For this review, take the finished solid that the model builds, in its own axes (mm). Give positions to 0.01 mm unless a question says otherwise; leave off trailing zeros. Write each loop counter-clockwise with the first axis right and the second up, starting at its lowest first coordinate (ties: lowest second). Pieces come first, ordered by that corner, then holes.
1) We need section C-C on x = 4.75. Give the boundary of the cut face in (y, z), and give its area (3 significant figures).
2) For P1, Ø1.5, axis at x = 0.5, z = 62, coming from the -Y side; P2, Ø2, axis at x = -5, z = 26.5, coming from the -Y side; P3, Ø1.8, axis at x = 0, y = -0.6, coming from the -Z side; P4, Ø2.5, axis at x = 0, z = 35.5, coming from the +Y side, all flat-tipped, find the tip position at first contact; note any pin that passes through.
3) We need section A-A on z = 35.5. Give the boundary of the cut face in (x, y).
4) We need section D-D on y = 1.25. Give the boundary of the cut face in (x, z).
5) We need section B-B on z = 45. Give the boundary of the cut face in (x, y).
6) Wall thickness on line 1 along Y through (x, z) = (0, 60.05) (3 decimals); line 2 along X through (y, z) = (-0.75, 54); line 3 along Z through (x, y) = (-1, -1): over which ranges is each line inside the solid? List them lowest first.
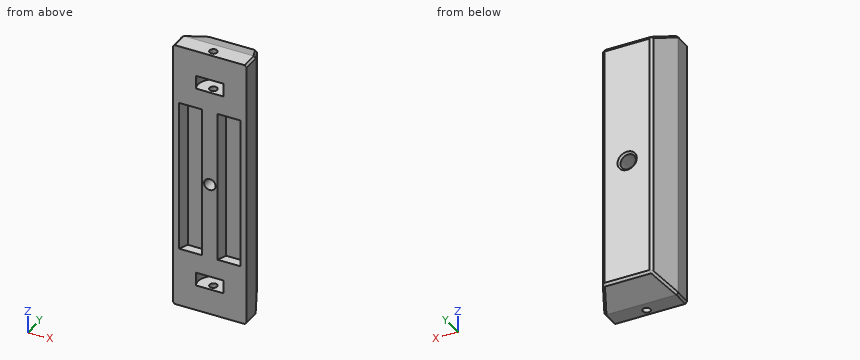
from build123d import *

# Parameters (mm, degrees)
EXTRUDE_1_DEPTH     = 71
CUT_EXTRUDE_1_DEPTH = 75.103710772
SKETCH_3_W          = 18.218739558
SKETCH_3_H          = 4.354088086
EXTRUDE_3_DEPTH     = 15.5
SKETCH_4_R          = 0.995
CUT_EXTRUDE_2_DEPTH = 12
SKETCH_5_W          = 4
SKETCH_5_H          = 3.5
SKETCH_6_R          = 1.5
CUT_EXTRUDE_3_DEPTH = 73.548604312
SKETCH_7_R          = 2.01
CUT_EXTRUDE_4_DEPTH = 5
CHAMFER_2_SIZE      = 0.5


with BuildPart() as part:
    # ｽｹｯﾁ1 → ﾎﾞｽ - 押し出し1 (new body)
    with BuildSketch(Plane.XY):
        Polygon((-6.990630221, 0), (-3.009369779, 0), (-1.990630221, -2.4), (1.990630221, -2.4), (3.009369779, 0), (6.990630221, 0), (8.009369779, -2.4), (9.609369779, -2.4), (9.609369779, 2), (6.345216172, 9), (-6.345216172, 9), (-9.609369779, 2), (-9.609369779, -2.4), (-8.009369779, -2.4), align=None)
    extrude(amount=EXTRUDE_1_DEPTH)

    # ｽｹｯﾁ2 → ｶｯﾄ - 押し出し1 (cut, through all)
    with BuildSketch(Plane(origin=(9.609369779, 0, 0), x_dir=(0, 0, -1), z_dir=(1, 0, 0))):
        Polygon((-71, 2), (-67.735846393, 9), (-71, 9), align=None)
        Polygon((-3.264153607, 9), (0, 9), (0, 2), align=None)
    extrude(amount=-CUT_EXTRUDE_1_DEPTH, mode=Mode.SUBTRACT)

    # 面取り1
    # the kernel refuses this chamfer: 0.5 mm, written as the material it takes off along each edge
    with BuildSketch(Plane(origin=(-6.138482875, 8.697897404, 3.470886905), x_dir=(0.1959067162203001, 0.5268881046463136, 0.8270486586180973), z_dir=(-0.41632572739388224, 0.8082980746110386, -0.4163257273938792)), Plane(origin=(6.138482875, 8.697897404, 3.470886905), x_dir=(-0.8270486586180952, 0.5268881046463165, 0.19590671622030123), z_dir=(0.4163257273938833, 0.8082980746110385, -0.41632572739387846))) as chamfer_1_piece_1:
        Polygon((-0.400884159, 0.228990916), (0.459173014, 0.228990916), (-0.058288855, -0.457981831), align=None)
    extrude(amount=0.4579583, mode=Mode.SUBTRACT)
    with BuildSketch(Plane(origin=(-6.138482875, 8.697897404, 67.529113095), x_dir=(-0.19590671622031064, -0.5268881046463169, 0.8270486586180926), z_dir=(-0.416325727393884, 0.808298074611038, 0.41632572739387863))) as chamfer_1_piece_2:
        Polygon((-0.459173014, 0.228990916), (0.400884159, 0.228990916), (0.058288855, -0.457981831), align=None)
    extrude(amount=0.4579583, mode=Mode.SUBTRACT)
    with BuildSketch(Plane(origin=(6.138482875, 8.697897404, 67.529113095), x_dir=(-0.8270486586180955, 0.5268881046463167, -0.19590671622029923), z_dir=(0.4163257273938827, 0.8082980746110371, 0.4163257273938819))) as chamfer_1_piece_3:
        Polygon((-0.400884159, -0.228990916), (0.459173014, -0.228990916), (-0.058288855, 0.457981831), align=None)
    extrude(amount=0.4579583, mode=Mode.SUBTRACT)
    with BuildSketch(Plane(origin=(9.609369779, -3.685841494, 71), x_dir=(-0.999621916911297, 0, 0.0274958766105822), z_dir=(0, 1, 0)), Plane(origin=(-9.609369779, 3.285841494, 71), x_dir=(0.999621916911297, 0, 0.0274958766105822), z_dir=(0, -1, 0))) as chamfer_1_piece_4:
        with BuildLine():
            Line((0.514336598, 0), (-0.028273577, -0.513558897))
            Line((-0.028273577, -0.513558897), (-0.038269797, -0.513283938))
            ThreePointArc((-0.038269797, -0.513283938), (-0.017064614, -0.256698915), (-0.009996219, 0.000274959))
            Line((-0.009996219, 0.000274959), (0.000274959, 0.009996219))
            ThreePointArc((0.000274959, 0.009996219), (0.257248832, 0.002927825), (0.514611556, 0.009996219))
            Line((0.514611556, 0.009996219), (0.514336598, 0))
        make_face()
    extrude(amount=6.971682988, mode=Mode.SUBTRACT)
    with BuildSketch(Plane(origin=(-9.609369779, 3.285841494, 0), x_dir=(0.9996219169112968, 0, -0.02749587661058639), z_dir=(0, -1, 0)), Plane(origin=(9.609369779, -3.685841494, 0), x_dir=(-0.9996219169112968, 0, -0.02749587661058639), z_dir=(0, 1, 0))) as chamfer_1_piece_5:
        with BuildLine():
            Line((0.514336598, 0), (-0.028273577, 0.513558897))
            Line((-0.028273577, 0.513558897), (-0.038269797, 0.513283938))
            ThreePointArc((-0.038269797, 0.513283938), (-0.017064614, 0.256698915), (-0.009996219, -0.000274959))
            Line((-0.009996219, -0.000274959), (0.000274959, -0.009996219))
            ThreePointArc((0.000274959, -0.009996219), (0.257248832, -0.002927825), (0.514611556, -0.009996219))
            Line((0.514611556, -0.009996219), (0.514336598, 0))
        make_face()
    extrude(amount=6.971682988, mode=Mode.SUBTRACT)
    with BuildSketch(Plane(origin=(-6.345216172, 9, 1.971704795), x_dir=(-0.441365564598093, -0.897327386401979, 0), z_dir=(0, 0, 1))) as chamfer_1_piece_6:
        with BuildLine():
            Line((0.516979525, 0), (-0.237770334, 0.459056747))
            Line((-0.237770334, 0.459056747), (-0.246743608, 0.454643091))
            ThreePointArc((-0.246743608, 0.454643091), (-0.123037104, 0.227486173), (-0.008973274, -0.004413656))
            Line((-0.008973274, -0.004413656), (0.000207861, -0.009997839))
            ThreePointArc((0.000207861, -0.009997839), (0.25858594, -0.004626004), (0.517187386, -0.009997839))
            Line((0.517187386, -0.009997839), (0.516979525, 0))
        make_face()
    extrude(amount=67.056590409, mode=Mode.SUBTRACT)
    with BuildSketch(Plane(origin=(6.345216172, 9, 1.971704795), x_dir=(0.441365564598093, -0.897327386401979, 0), z_dir=(0, 0, 1))) as chamfer_1_piece_7:
        with BuildLine():
            Line((0.516979525, 0), (-0.237770334, -0.459056747))
            Line((-0.237770334, -0.459056747), (-0.246743608, -0.454643091))
            ThreePointArc((-0.246743608, -0.454643091), (-0.123037104, -0.227486173), (-0.008973274, 0.004413656))
            Line((-0.008973274, 0.004413656), (0.000207861, 0.009997839))
            ThreePointArc((0.000207861, 0.009997839), (0.25858594, 0.004626004), (0.517187386, 0.009997839))
            Line((0.517187386, 0.009997839), (0.516979525, 0))
        make_face()
    extrude(amount=67.056590409, mode=Mode.SUBTRACT)
    with BuildSketch(Plane(origin=(7.637664984, 9, 67.735846393), x_dir=(0, -0.8973273864019788, 0.441365564598093), z_dir=(-1, 0, 0))) as chamfer_1_piece_8:
        with BuildLine():
            Line((0.516979525, 0), (-0.237770334, -0.459056747))
            Line((-0.237770334, -0.459056747), (-0.246743608, -0.454643091))
            ThreePointArc((-0.246743608, -0.454643091), (-0.123037104, -0.227486173), (-0.008973274, 0.004413656))
            Line((-0.008973274, 0.004413656), (0.000207861, 0.009997839))
            ThreePointArc((0.000207861, 0.009997839), (0.25858594, 0.004626004), (0.517187386, 0.009997839))
            Line((0.517187386, 0.009997839), (0.516979525, 0))
        make_face()
    extrude(amount=15.275329968, mode=Mode.SUBTRACT)
    with BuildSketch(Plane(origin=(5.843517245, 10.075896822, 67.234147465), x_dir=(-0.9208340423276119, -0.34219239318368305, 0.1870000869994816), z_dir=(0.38928162063502697, -0.8348171294789895, 0.3892816206350193)), Plane(origin=(-10.111068707, 0.924103178, 71.501698928), x_dir=(0.9208340423276127, -0.3421923931836955, 0.1870000869994551), z_dir=(0.3892816206350268, 0.8348171294789896, -0.38928162063501937))) as chamfer_1_piece_9:
        with BuildLine():
            Line((0.515512576, 0), (-0.117174183, 0.502019349))
            Line((-0.117174183, 0.502019349), (-0.126965941, 0.499989208))
            ThreePointArc((-0.126965941, 0.499989208), (-0.062103739, 0.250280562), (-0.009791758, -0.002030141))
            Line((-0.009791758, -0.002030141), (0.000248629, -0.009996909))
            ThreePointArc((0.000248629, -0.009996909), (0.257845581, -0.003590326), (0.515761205, -0.009996909))
            Line((0.515761205, -0.009996909), (0.515512576, 0))
        make_face()
    extrude(amount=10.962632798, mode=Mode.SUBTRACT)
    with BuildSketch(Plane(origin=(5.843517245, 10.075896822, 3.765852535), x_dir=(-0.9208340423276121, -0.3421923931836904, -0.18700008699946713), z_dir=(0.3892816206350273, -0.8348171294789902, -0.38928162063501737)), Plane(origin=(-10.111068707, 0.924103178, -0.501698928), x_dir=(0.9208340423276121, -0.3421923931836903, -0.18700008699946674), z_dir=(0.38928162063502714, 0.8348171294789903, 0.38928162063501737))) as chamfer_1_piece_10:
        with BuildLine():
            Line((0.515512576, 0), (-0.117174183, -0.502019349))
            Line((-0.117174183, -0.502019349), (-0.126965941, -0.499989208))
            ThreePointArc((-0.126965941, -0.499989208), (-0.062103739, -0.250280562), (-0.009791758, 0.002030141))
            Line((-0.009791758, 0.002030141), (0.000248629, 0.009996909))
            ThreePointArc((0.000248629, 0.009996909), (0.257845581, 0.003590326), (0.515761205, 0.009996909))
            Line((0.515761205, 0.009996909), (0.515512576, 0))
        make_face()
    extrude(amount=10.962632798, mode=Mode.SUBTRACT)
    with BuildSketch(Plane(origin=(7.637664984, 9, 3.264153607), x_dir=(0, -0.8973273864019832, -0.4413655645980848), z_dir=(-1, 0, 0))) as chamfer_1_piece_11:
        with BuildLine():
            Line((0.516979525, 0), (-0.237770334, 0.459056747))
            Line((-0.237770334, 0.459056747), (-0.246743608, 0.454643091))
            ThreePointArc((-0.246743608, 0.454643091), (-0.123037104, 0.227486173), (-0.008973274, -0.004413656))
            Line((-0.008973274, -0.004413656), (0.000207861, -0.009997839))
            ThreePointArc((0.000207861, -0.009997839), (0.25858594, -0.004626004), (0.517187386, -0.009997839))
            Line((0.517187386, -0.009997839), (0.516979525, 0))
        make_face()
    extrude(amount=15.275329968, mode=Mode.SUBTRACT)

    # ｽｹｯﾁ3 → ﾎﾞｽ - 押し出し3 (add)
    with BuildSketch(Plane.XY.offset(71)):
        with Locations((0, -0.222955957)):
            Rectangle(SKETCH_3_W, SKETCH_3_H)
    extrude_3 = extrude(amount=-EXTRUDE_3_DEPTH)

    # ｽｹｯﾁ4 → ｶｯﾄ - 押し出し2 (cut)
    with BuildSketch(Plane.XY.offset(71)):
        with Locations((0, -0.6)):
            Circle(SKETCH_4_R)
    cut_extrude_2 = extrude(amount=-CUT_EXTRUDE_2_DEPTH, mode=Mode.SUBTRACT)

    # ﾐﾗｰ1: ﾎﾞｽ - 押し出し3, ｶｯﾄ - 押し出し2 across plane
    add(extrude_3.mirror(Plane(origin=(0, 0, 35.5), x_dir=(1, 0, 0), z_dir=(0, 0, -1))))
    add(cut_extrude_2.mirror(Plane(origin=(0, 0, 35.5), x_dir=(1, 0, 0), z_dir=(0, 0, -1))), mode=Mode.SUBTRACT)

    # ｽｹｯﾁ5 → ｶｯﾄ - 回転1 (revolve, cut)
    with BuildSketch(Plane(origin=(0, -0.6, 0), x_dir=(1, 0, 0), z_dir=(0, 1, 0))):
        with Locations((2, -62.5)):
            Rectangle(SKETCH_5_W, SKETCH_5_H)
        with Locations((2, -8.5)):
            Rectangle(SKETCH_5_W, SKETCH_5_H)
    revolve(axis=Axis((0, -0.6, 59), (0, 0, 1)), mode=Mode.SUBTRACT)

    # ｽｹｯﾁ6 → ｶｯﾄ - 押し出し3 (cut, through all)
    with BuildSketch(Plane.XZ.offset(2.4)):
        with Locations(Location((0, 35.5, 0), (0, 0, 270))):
            Circle(SKETCH_6_R)
    extrude(amount=-CUT_EXTRUDE_3_DEPTH, mode=Mode.SUBTRACT)

    # ｽｹｯﾁ7 → ｶｯﾄ - 押し出し4 (cut)
    with BuildSketch(Plane(origin=(0, 9, 0), x_dir=(1, 0, 0), z_dir=(0, 1, 0))):
        with Locations(Location((0, -35.5, 0), (0, 0, 180))):
            Circle(SKETCH_7_R)
    extrude(amount=-CUT_EXTRUDE_4_DEPTH, mode=Mode.SUBTRACT)

    # 面取り2
    chamfer_2_edges = [part.edges().sort_by_distance(p)[0] for p in [
        (2.01, 9, 35.5),
    ]]
    chamfer(chamfer_2_edges, length=CHAMFER_2_SIZE)


solid = part.part
Results list:
1. outline: (-2.4, 0) - (2, 0) - (8.55, 3.05) - (9, 3.76) - (9, 67.24) - (8.55, 67.95) - (2, 71) - (-2.4, 71) - (-2.4, 55.5) - (0, 55.5) - (0, 15.5) - (-2.4, 15.5) - close
1. area: 690 mm2
2. P1: stops at y = 3.2
2. P2: stops at y = 0
2. P3: stops at z = 12
2. P4: passes through
3. outline: (-9.61, -2.4) - (-8.01, -2.4) - (-6.99, 0) - (-3.01, 0) - (-1.99, -2.4) - (-1.5, -2.4) - (-1.5, 4) - (-2.01, 4) - (-2.01, 8.5) - (-2.51, 9) - (-5.85, 9) - (-6.56, 8.55) - (-9.61, 2) - close; (1.5, -2.4) - (1.99, -2.4) - (3.01, 0) - (6.99, 0) - (8.01, -2.4) - (9.61, -2.4) - (9.61, 2) - (6.56, 8.55) - (5.85, 9) - (2.51, 9) - (2.01, 8.5) - (2.01, 4) - (1.5, 4) - close
4. outline: (-9.61, 0.5) - (-9.11, 0) - (9.11, 0) - (9.61, 0.5) - (9.61, 70.5) - (9.11, 71) - (-9.11, 71) - (-9.61, 70.5) - close; hole (-3.55, 6.75) - (3.55, 6.75) - (3.55, 10.25) - (-3.55, 10.25) - close; hole (-3.55, 60.75) - (3.55, 60.75) - (3.55, 64.25) - (-3.55, 64.25) - close; hole circle Ø3 at (0, 35.5)
5. outline: (-9.61, -2.4) - (-8.01, -2.4) - (-6.99, 0) - (-3.01, 0) - (-1.99, -2.4) - (1.99, -2.4) - (3.01, 0) - (6.99, 0) - (8.01, -2.4) - (9.61, -2.4) - (9.61, 2) - (6.56, 8.55) - (5.85, 9) - (-5.85, 9) - (-6.56, 8.55) - (-9.61, 2) - close
6. line 1: y = -2.4 to -1.595, 0.395 to 9
6. line 2: x = -9.61 to -7.31, -2.69 to 2.69, 7.31 to 9.61
6. line 3: z = 0 to 6.75, 10.25 to 34.38, 36.62 to 60.75, 64.25 to 71
